```python
from build123d import *

# Parameters (mm, degrees)
SKETCH1_W                                       = 25.4
SKETCH1_H                                       = 6
SKETCH2_R                                       = 15
BOSS_EXTRUDE1_DEPTH                             = 56.2
CUT_EXTRUDE1_DEPTH                              = 24.1
SKETCH5_W                                       = 1.25
SKETCH5_H                                       = 16.341500105
M3X0_5_TAPPED_HOLE1_D                           = 2.5
M3X0_5_TAPPED_HOLE1_DEPTH                       = 12
M3X0_5_TAPPED_HOLE1_TIP                         = 0.751075774
CSK_FOR_M4_FLAT_HEAD_MACHINE_SCREW1_D           = 4.8
CSK_FOR_M4_FLAT_HEAD_MACHINE_SCREW1_CSINK_D     = 9.4
CSK_FOR_M4_FLAT_HEAD_MACHINE_SCREW1_CSINK_ANGLE = 90


with BuildPart() as part:
    # Sketch1 → Revolve1 (revolve)
    with BuildSketch(Plane.XZ, mode=Mode.PRIVATE) as revolve1_sk:
        with Locations((12.7, 58.54)):
            Rectangle(SKETCH1_W, SKETCH1_H)
    revolve(revolve1_sk.sketch.rotate(Axis((0, 0, 61.54), (0, 0, -1)), 180), axis=Axis((0, 0, 61.54), (0, 0, -1)))

    # Sketch2 → Boss-Extrude1 (add)
    with BuildSketch(Plane(origin=(0, 0, 55.54), x_dir=(-1, 0, 0), z_dir=(0, 0, -1))):
        Circle(SKETCH2_R)
    extrude(amount=BOSS_EXTRUDE1_DEPTH)

    # Sketch3 → Cut-Extrude1 (cut)
    with BuildSketch(Plane(origin=(0, 0, -0.66), x_dir=(-1, 0, 0), z_dir=(0, 0, -1))):
        with BuildLine():
            Line((2.5, 9.058499895), (-2.5, 9.058499895))
            Line((-2.5, 9.058499895), (-2.5, 6.549481518))
            ThreePointArc((-2.5, 6.549481518), (0, 7.0104), (2.5, 6.549481518))
            Line((2.5, 6.549481518), (2.5, 9.058499895))
        make_face()
    extrude(amount=-CUT_EXTRUDE1_DEPTH, mode=Mode.SUBTRACT)

    # Sketch4 → Cut-Revolve1 (revolve, cut)
    with BuildSketch(Plane(origin=(0, 0, 0), x_dir=(1, 0, 0), z_dir=(0, 1, 0))):
        Polygon((7.0104, 0.66), (0, 0.66), (0, -61.54), (10.3124, -61.54), (10.3124, -23.44), (7.0104, -23.44), align=None)
    revolve(axis=Axis((0, 0, -0.66), (0, 0, 1)), mode=Mode.SUBTRACT)

    # Sketch5 → M3x0.5 Tapped Hole2 (revolve, cut)
    with BuildSketch(Plane(origin=(0, 9.058499895, 20.422), x_dir=(0, 0, -1), z_dir=(1, 0, 0))):
        with Locations((0.625, 8.170750053)):
            Rectangle(SKETCH5_W, SKETCH5_H)
    revolve(axis=Axis((0, 2.708499895, 20.422), (0, 1, 0)), mode=Mode.SUBTRACT)

    # M3x0.5 Tapped Hole1
    with Locations(Plane(origin=(0, 0, -0.66), x_dir=(-1, 0, 0), z_dir=(0, 0, -1))):
        with Locations((-11.5, 0), (-5.75, -9.959292144), (5.75, -9.959292144), (11.5, 0), (5.75, 9.959292144), (-5.75, 9.959292144)):
            Hole(M3X0_5_TAPPED_HOLE1_D / 2, depth=M3X0_5_TAPPED_HOLE1_DEPTH)
            with Locations((0, 0, -(M3X0_5_TAPPED_HOLE1_DEPTH + M3X0_5_TAPPED_HOLE1_TIP / 2))):  # 118° drill point
                Cone(0, M3X0_5_TAPPED_HOLE1_D / 2, M3X0_5_TAPPED_HOLE1_TIP, mode=Mode.SUBTRACT)

    # CSK for M4 Flat Head Machine Screw1 (through all)
    with Locations(Plane.XY.offset(61.54)):
        with Locations((0, 20.4), (14.424978336, 14.424978336), (20.4, 0), (14.424978336, -14.424978336), (0, -20.4), (-14.424978336, -14.424978336), (-20.4, 0), (-14.424978336, 14.424978336)):
            CounterSinkHole(CSK_FOR_M4_FLAT_HEAD_MACHINE_SCREW1_D / 2, CSK_FOR_M4_FLAT_HEAD_MACHINE_SCREW1_CSINK_D / 2, counter_sink_angle=CSK_FOR_M4_FLAT_HEAD_MACHINE_SCREW1_CSINK_ANGLE)


solid = part.part
```
Geometry: final body of the model. Coordinates: model frame, mm. A direction names the side the tool comes from. Round coordinates to 2 decimals unless told otherwise and drop trailing zeros. Write each loop counter-clockwise with the first axis right and the second up, starting at its lowest first coordinate (ties: lowest second). Pieces come first, ordered by that corner, then holes. Notation, with made-up numbers: M -15,-40 L 27,-40 A12 cw 27,-23 Z; hole C 45,86 d5. An arc over 180 degrees is marked long. Answer in a Markdown table with one row per item. Add a question column.
(1) Reachability of faces 1 (the face through (0, 9.058, 11)), 2 (the face through (2, -7, 23.44)), 3 (the face through (-11.7, -0.08, 11.96)) from +Z, -Z, +X, -X, +Y, -Y: full face, straight path, thin tool, end or side. Return the list, or none.
(2) Cut plane A-A, the plane x = 0. Give the number of separate pieces and of enclosed holes in the cut face, then the cut area to 3 significant figures.
(3) Cut plane C-C, the plane z = 8. Return the cut outline in (x, y), then the cut area to 3 significant figures.
(4) Draft query along Y for faces 4 (the face through (-5.59, -9.81, 11.96)), 5 (the face through (14.985, 0.66, 27.833)), 6 (the face through (-7, -10, 5)), 7 (the face through (-0.05, 12.07, 21.67)). Return one class per face: pulls with the +Y half, pulls with the -Y half, needs draft (parallel to the pull), parting line crosses it, or undercut.
(5) Contact query for flat-ended pins moving along their axis: pin 1 (7.5 mm diameter, centred on x = 20.4, y = 0, fed in from -Z); pin 2 (16.5 mm diameter, centred on x = 0, y = 0, fed in from +Z); pin 3 (8 mm diameter, centred on x = -0.5, z = 29, fed in from +Y). Output: stop coordinate, or through.
(6) Ray query, L1, parallel to Z at x = 21, y = 8.5; L2, parallel to Y at x = 11.5, z = 8.5; L3, parallel to Y at x = 2.5, z = 46. Return the intervals inside material, ascending.
(7) Cut plane B-B, the plane z = 17. Return the cut outline in (x, y), then the cut area to 3 significant figures.
(8) Cut plane D-D, the plane x = 20.4. Return the cut outline in (y, z), then the cut area to 3 significant figures.
Established:
| question | item | result |
|---|---|---|
| 1 | face 1 | +Z, -Z |
| 1 | face 2 | +Z |
| 1 | face 3 | -Z |
| 2 | separate pieces | 5 |
| 2 | enclosed holes | 0 |
| 2 | area | 735 mm² |
| 3 | outline | C 0,0 d30; hole C -11.5,0 d2.5; hole C -5.75,-9.96 d2.5; hole C -5.75,9.96 d2.5; hole M -2.5,6.55 A7.01 ccw long 2.5,6.55 L 2.5,9.06 L -2.5,9.06 Z; hole C 5.75,-9.96 d2.5; hole C 5.75,9.96 d2.5; hole C 11.5,0 d2.5 |
| 3 | area | 512 mm² |
| 4 | face 4 | undercut |
| 4 | face 5 | parting line crosses it |
| 4 | face 6 | undercut |
| 4 | face 7 | needs draft |
| 5 | pin 1 | z = 55.54 |
| 5 | pin 2 | z = 23.44 |
| 5 | pin 3 | y = 15 |
| 6 | L1 | 55.54 to 61.54 |
| 6 | L2 | -9.63 to -1.25, 1.25 to 9.63 |
| 6 | L3 | -14.79 to -10, 10 to 14.79 |
| 7 | outline | C 0,0 d30; hole M -2.5,6.55 A7.01 ccw long 2.5,6.55 L 2.5,9.06 L -2.5,9.06 Z |
| 7 | area | 541 mm² |
| 8 | outline | M -15.13,55.54 L -2.4,55.54 L -2.4,59.24 L -4.7,61.54 L -15.13,61.54 Z; M 2.4,55.54 L 15.13,55.54 L 15.13,61.54 L 4.7,61.54 L 2.4,59.24 Z |
| 8 | area | 148 mm² |
